from build123d import *

# Parameters (mm, degrees)
F0_W      = 600.075
F0_H      = 1450.975
F1_DEPTH  = 274.6375
F2_T      = -50.8
F4_DEPTH  = 22.225
F5_W      = 600.075
F5_H      = 1.5875
F6_DEPTH  = 57.15
F7_W      = 600.075
F7_H      = 88.9
F8_DEPTH  = 1.5875
F10_DEPTH = 600.075


with BuildPart() as f1:
    # F0 (on Front) → F1 (new body, symmetric)
    with BuildSketch(Plane.XZ):
        Rectangle(F0_W, F0_H)
    extrude(amount=F1_DEPTH, both=True)

    # F2
    f2_openings = [f1.faces().sort_by_distance(p)[0] for p in [
        (0, -274.6375, 0),
    ]]
    offset(amount=F2_T, openings=f2_openings)

    # F3 (on face) → F4 (join)
    with BuildSketch(Plane(origin=(0, 0, -725.4875), x_dir=(1, 0, 0), z_dir=(0, 0, -1))):
        with BuildLine():
            ThreePointArc((-250.825, 241.3), (-277.92532, 252.52532), (-266.7, 225.425))
            Line((-266.7, 225.425), (-266.7, 241.3))
            Line((-266.7, 241.3), (-250.825, 241.3))
        make_face()
        with BuildLine():
            Line((-266.7, 241.3), (-266.7, 225.425))
            ThreePointArc((-266.7, 225.425), (-255.47468, 230.07468), (-250.825, 241.3))
            Line((-250.825, 241.3), (-266.7, 241.3))
        make_face()
        with BuildLine():
            ThreePointArc((250.825, 241.3), (255.47468, 230.07468), (266.7, 225.425))
            Line((266.7, 225.425), (266.7, 241.3))
            Line((266.7, 241.3), (250.825, 241.3))
        make_face()
        with BuildLine():
            Line((266.7, 241.3), (266.7, 225.425))
            ThreePointArc((266.7, 225.425), (277.92532, 230.07468), (282.575, 241.3))
            ThreePointArc((282.575, 241.3), (266.7, 257.175), (250.825, 241.3))
            Line((250.825, 241.3), (266.7, 241.3))
        make_face()
        with BuildLine():
            ThreePointArc((266.7, -225.425), (255.47468, -230.07468), (250.825, -241.3))
            Line((250.825, -241.3), (266.7, -241.3))
            Line((266.7, -241.3), (266.7, -225.425))
        make_face()
        with BuildLine():
            Line((266.7, -241.3), (250.825, -241.3))
            ThreePointArc((250.825, -241.3), (266.7, -257.175), (282.575, -241.3))
            ThreePointArc((282.575, -241.3), (277.92532, -230.07468), (266.7, -225.425))
            Line((266.7, -225.425), (266.7, -241.3))
        make_face()
        with BuildLine():
            Line((-266.7, -241.3), (-250.825, -241.3))
            ThreePointArc((-250.825, -241.3), (-255.47468, -230.07468), (-266.7, -225.425))
            Line((-266.7, -225.425), (-266.7, -241.3))
        make_face()
        with BuildLine():
            ThreePointArc((-266.7, -225.425), (-277.92532, -252.52532), (-250.825, -241.3))
            Line((-250.825, -241.3), (-266.7, -241.3))
            Line((-266.7, -241.3), (-266.7, -225.425))
        make_face()
    extrude(amount=F4_DEPTH)

    # F5 (on face) → F6 (join)
    with BuildSketch(Plane.XZ.offset(274.6375)):
        with Locations((0, 718.34375)):
            Rectangle(F5_W, F5_H)
    extrude(amount=F6_DEPTH)

    # F7 (on face) → F8 (join)
    with BuildSketch(Plane.XY.offset(725.4875)):
        with Locations((0, -230.1875)):
            Rectangle(F7_W, F7_H)
    extrude(amount=F8_DEPTH)

    # F9 (on face) → F10 (join)
    with BuildSketch(Plane.YZ.offset(300.0375)):
        Polygon((-274.6375, 719.1375), (-274.6375, 727.075), (-283.236563, 719.1375), align=None)
    extrude(amount=-F10_DEPTH)


solid = f1.part
Build history of the part. All positions in model axes, mm. A direction names the side the tool comes from. Give positions to 0.01 mm unless a question says otherwise; leave off trailing zeros. Loops run counter-clockwise (first coordinate to the right, second up) from the corner with the lowest first, then second, coordinate; pieces in that order, holes last. Notation, with made-up numbers: (-18, 31.25) - (17, 31.25) arc R31 ccw to (17, 57.25) - close; hole circle Ø9 at (-21, 70). An arc over 180 degrees is marked (long way). Write item = value, one per line. Start each with the question number.
1) Pull direction X, two halves, no side cores. Call faces 5 (the flat face through (300.038, -33, 11)), 6 (the flat face through (-267, -242, -747.712)), 7 (the flat face through (-3, -29, -674.688)): +X half, -X half, draft (parallel to the pull), parting line (faces both ways), or undercut.
2) Band-saw the part on B-B on z = -623. Give the cut face in (x, y).
3) Drop flat-ended pins along their axis: pin 1 Ø0.8 at (x, z) = (-53.5, 726) entering from +Y; pin 2 Ø5 at (x, y) = (-75, 153) entering from -Z; pin 3 Ø17 at (x, y) = (-86.5, -299.5) entering from -Z. Give the stop position or say it passes through.
4) Tool access for faces 1 (the flat face through (-4, 41, 725.488)), 2 (the flat face through (-3, 223.837, 9)), 3 (the flat face through (-4, -307, 719.138)), 4 (the flat face through (-268, -274.638, 53)): list every direction of +Z, -Z, +X, -X, +Y, -Y with a clear straight run to the whole face (end or side of a thin tool).
5) Probe probe 1 along Z at (x, y) = (-160.5, -193.5) (1 decimal); probe 2 along X at (y, z) = (-245, -501); probe 3 along Z at (x, y) = (132.5, -91). List the from-to ranges inside material, lowest first. Write a range as from..to.
6) Band-saw the part on A-A on y = -1. Give the cut face in (x, z), plus the area to 3 significant figures.
Final values:
q1.face_5 = +X half
q1.face_6 = draft
q1.face_7 = undercut
q2.outline = (-300.04, -274.64) - (-249.24, -274.64) - (-249.24, 223.84) - (249.24, 223.84) - (249.24, -274.64) - (300.04, -274.64) - (300.04, 274.64) - (-300.04, 274.64) - close
q3.pin_1 = -185.74
q3.pin_2 = -725.49
q3.pin_3 = 717.55
q4.face_1 = +Z, +X, -X, +Y
q4.face_2 = -Y
q4.face_3 = +Z, +X, -X, -Y
q4.face_4 = -Z, +X, -X, -Y
q5.probe_1 = -725.5..-674.7, 674.7..727.1
q5.probe_2 = -300.04..-249.24, 249.24..300.04
q5.probe_3 = -725.49..-674.69, 674.69..725.49
q6.outline = (-300.04, -725.49) - (300.04, -725.49) - (300.04, 725.49) - (-300.04, 725.49) - close; hole (-249.24, -674.69) - (249.24, -674.69) - (249.24, 674.69) - (-249.24, 674.69) - close
q6.area = 198,000 mm²
